Verification items for the finished model (mm, model axes). A direction names the side the tool comes from. Round coordinates to 2 decimals unless told otherwise and drop trailing zeros. Order: outer loops, then holes, each group sorted by start corner. A loop starts at its lowest first (then second) coordinate and runs counter-clockwise, first axis right, second up. Notation, with made-up numbers: M 75.25,36.5 L 130.25,36.5 A35 cw 130.25,70.5 Z; hole C 7.25,37 d5. An arc over 180 degrees is marked long. Return JSON: item names as keys, results as strings. Group by question number.
from build123d import *

# Parameters (mm, degrees)
F0_W         = 100
F0_H         = 100
F1_DEPTH     = 0.7
F2_W         = 96.2
F2_H         = 97.5
F2_W_2       = 90.8
F2_H_2       = 92.1
F3_DEPTH     = 1.9
F5_DEPTH     = 3
F6_T1_DEPTH  = 90.8
F6_T3_DEPTH  = 99.8150489639
F6_T9_DEPTH  = 99.8150489639
F6_T15_DEPTH = 98.5150489639
F6_T24_DEPTH = 99.8150489639
F6_T30_DEPTH = 98.5150489639


# Not quite as in the source:
# - a fillet or chamfer that OpenCascade refuses, or shapes differently, is made with other operations: its cross-section is extruded or revolved along the edge and cut away or added


with BuildPart() as f1:
    # F0 (on Top) → F1 (new body)
    with BuildSketch(Plane.XY):
        Rectangle(F0_W, F0_H)
    extrude(amount=F1_DEPTH)

    # F2 (on face) → F3 (join)
    with BuildSketch(Plane.XY.offset(0.7)):
        with Locations((0, -1.25)):
            Rectangle(F2_W, F2_H)
        with Locations((0, -1.25)):
            Rectangle(F2_W_2, F2_H_2, mode=Mode.SUBTRACT)
    extrude(amount=F3_DEPTH)

    # F4 (on face) → F5 (join)
    with BuildSketch(Plane.XY.offset(2.6)):
        Polygon((-48.1, -47.3), (-45.4, -47.3), (-45.4, 44.8), (45.4, 44.8), (45.4, -47.3), (48.1, -47.3), (48.1, 47.5), (-48.1, 47.5), align=None)
    extrude(amount=F5_DEPTH)

    # F6: chamfer of 3 on 3 edges, made by hand

    # F6_s2 → F6_t1 (cut)
    with BuildSketch(Plane.YZ.offset(-45.4)):
        Polygon((44.8, 2.6), (47.8, 5.6), (44.8, 5.6), align=None)
    extrude(amount=F6_T1_DEPTH, mode=Mode.SUBTRACT)

    # F6_s4 → F6_t3 (cut)
    with BuildSketch(Plane.XZ.offset(-44.8)):
        Polygon((-45.4, 2.6), (-48.4, 5.6), (-45.4, 5.6), align=None)
        Polygon((45.4, 2.6), (48.4, 5.6), (45.4, 5.6), align=None)
    extrude(amount=F6_T3_DEPTH, mode=Mode.SUBTRACT)


with BuildPart() as f6_tool7:
    # F6_s8 → F6_t9 (new body)
    with BuildSketch(Plane.XZ.offset(47.3)):
        Polygon((-45.4, 2.6), (-48.4, 5.6), (-45.4, 5.6), align=None)
    extrude(amount=-F6_T9_DEPTH)

    split(bisect_by=Plane.YZ.offset(-48.1), keep=Keep.TOP)

    split(bisect_by=Plane.XZ.offset(-44.8), keep=Keep.BOTTOM)

    split(bisect_by=Plane.XZ.offset(-47.5), keep=Keep.TOP)


with BuildPart() as f6_tool13:
    # F6_s14 → F6_t15 (new body)
    with BuildSketch(Plane.YZ.offset(-53.1150489639)):
        Polygon((44.8, 2.6), (47.8, 5.6), (44.8, 5.6), align=None)
    extrude(amount=F6_T15_DEPTH)

    split(bisect_by=Plane.YZ.offset(-48.1), keep=Keep.TOP)

    split(bisect_by=Plane.YZ.offset(-45.4), keep=Keep.BOTTOM)

    split(bisect_by=Plane.XZ.offset(-47.5), keep=Keep.TOP)


with BuildPart() as f6_tool7_1:
    add(f6_tool7.part)

    # F6_t19: intersect F6_tool13
    add(f6_tool13.part, mode=Mode.INTERSECT)


with BuildPart() as f1_1:
    add(f1.part)

    # F6_t5: cut F6_tool7
    add(f6_tool7_1.part, mode=Mode.SUBTRACT)


with BuildPart() as f6_tool22:
    # F6_s23 → F6_t24 (new body)
    with BuildSketch(Plane.XZ.offset(-52.5150489639)):
        Polygon((45.4, 2.6), (48.4, 5.6), (45.4, 5.6), align=None)
    extrude(amount=F6_T24_DEPTH)

    split(bisect_by=Plane.XZ.offset(-44.8), keep=Keep.BOTTOM)

    split(bisect_by=Plane.XZ.offset(-47.5), keep=Keep.TOP)

    split(bisect_by=Plane.YZ.offset(48.1), keep=Keep.BOTTOM)


with BuildPart() as f6_tool28:
    # F6_s29 → F6_t30 (new body)
    with BuildSketch(Plane.YZ.offset(-45.4)):
        Polygon((44.8, 2.6), (47.8, 5.6), (44.8, 5.6), align=None)
    extrude(amount=F6_T30_DEPTH)

    split(bisect_by=Plane.YZ.offset(45.4), keep=Keep.TOP)

    split(bisect_by=Plane.XZ.offset(-47.5), keep=Keep.TOP)

    split(bisect_by=Plane.YZ.offset(48.1), keep=Keep.BOTTOM)


with BuildPart() as f6_tool22_1:
    add(f6_tool22.part)

    # F6_t34: intersect F6_tool28
    add(f6_tool28.part, mode=Mode.INTERSECT)


with BuildPart() as f1_2:
    add(f1_1.part)

    # F6_t20: cut F6_tool22
    add(f6_tool22_1.part, mode=Mode.SUBTRACT)


solid = f1_2.part
1. Cross-section at A-A (z = 4.25). Enter the section's corners in (x, y), plus the area to 3 significant figures.
2. Go/stop test with flat-tipped pins: pin 1 (1 mm diameter, centred on y = 2.5, z = 3, fed in from +X); pin 2 (2 mm diameter, centred on x = 19, z = 2, fed in from +Y); pin 3 (2 mm diameter, centred on x = 47, z = 4, fed in from -Y). Record where each tip stops, or that it passes through.
3. Draft check along Y on faces 1 (the face through (-1, -1, 0.7)), 2 (the face through (-48.4, 22.5, 0.7)), 3 (the face through (47, -47.3, 3)). Enter one of: +Y half, -Y half, draft (parallel to the pull), parting line (faces both ways), or undercut.
4. Cross-section at B-B (y = 7). Enter the section's corners in (x, z), plus the area to 4 significant figures.
5. Thickness scan on line 1 along X through (y, z) = (-17, 1.4); line 2 along Y through (x, z) = (9, 2.5); line 3 along Z through (x, y) = (30, 19.5). Record the ranges inside material, lowest first. Write a range as from..to.
6. Cross-section at C-C (x = -9.5). Enter the section's corners in (y, z).
7. Access from +Z, -Z, +X, -X, +Y, -Y to the whole of each face (thin tool, end or side, straight path). Record for faces 4 (the face through (-1, -49, 2.6)), 5 (the face through (1, 47.5, 3)), 6 (the face through (-48.1, -1, 3)), 7 (the face through (48.1, -2, 3)), 8 (the face through (46.7, 0.8, 3.9)).
Computed:
{
 "1": {"outline": "M -48.1,-47.3 L -47.05,-47.3 L -47.05,46.45 L 47.05,46.45 L 47.05,-47.3 L 48.1,-47.3 L 48.1,47.5 L -48.1,47.5 Z", "area": "298 mm²"},
 "2": {"pin 1": "stops at x = 48.1", "pin 2": "stops at y = 47.5", "pin 3": "stops at y = -47.3"},
 "3": {"face 1": "undercut", "face 2": "draft", "face 3": "-Y half"},
 "4": {"outline": "M -50,0 L 50,0 L 50,0.7 L 48.1,0.7 L 48.1,5.3 L 45.4,2.6 L 45.4,0.7 L -45.4,0.7 L -45.4,2.6 L -48.1,5.3 L -48.1,0.7 L -50,0.7 Z", "area": "87.55 mm²"},
 "5": {"line 1": "x = -48.1..-45.4, 45.4..48.1", "line 2": "y = -50..-47.3, 44.8..47.5", "line 3": "z = 0..0.7"},
 "6": {"outline": "M -50,0 L 50,0 L 50,0.7 L 47.5,0.7 L 47.5,5.3 L 44.8,2.6 L 44.8,0.7 L -47.3,0.7 L -47.3,2.6 L -50,2.6 Z"},
 "7": {"face 4": "+Z, +X, -X, -Y", "face 5": "+Z, +X, -X, +Y", "face 6": "+Z, -X, +Y, -Y", "face 7": "+Z, +X, +Y, -Y", "face 8": "+Z, -Y"}
}
